```python
from build123d import *

# Parameters (mm, degrees)
SKETCH1_W           = 40.2
SKETCH1_H           = 61.1
BOSS_EXTRUDE1_DEPTH = 41
CHAMFER1_SIZE       = 1
CHAMFER2_SIZE       = 1
SKETCH2_R           = 5
BOSS_EXTRUDE2_DEPTH = 1


with BuildPart() as part:
    # Sketch1 → Boss-Extrude1 (new body)
    with BuildSketch(Plane(origin=(0, 0, 0), x_dir=(1, 0, 0), z_dir=(0, 1, 0))):
        with Locations((20.1, 30.55)):
            Rectangle(SKETCH1_W, SKETCH1_H)
    extrude(amount=BOSS_EXTRUDE1_DEPTH)

    # Chamfer1
    chamfer1_edges = [part.edges().sort_by_distance(p)[0] for p in [
        (40.2, 41, -30.55),
        (20.1, 41, -61.1),
        (0, 41, -30.55),
        (20.1, 41, 0),
    ]]
    chamfer(chamfer1_edges, length=CHAMFER1_SIZE)

    # Chamfer2
    chamfer2_edges = [part.edges().sort_by_distance(p)[0] for p in [
        (20.1, 0, -61.1),
        (40.2, 0, -30.55),
        (20.1, 0, 0),
        (0, 0, -30.55),
    ]]
    chamfer(chamfer2_edges, length=CHAMFER2_SIZE)

    # Sketch2 → Boss-Extrude2 (add)
    with BuildSketch(Plane.XZ):
        with Locations(Location((20.1, -17.640972678, 0), (0, 0, 90))):
            Circle(SKETCH2_R)
    boss_extrude2 = extrude(amount=BOSS_EXTRUDE2_DEPTH)

    # Mirror1: Boss-Extrude2 across plane
    add(boss_extrude2.mirror(Plane.ZX.offset(20.5)))


solid = part.part
```
The model under review builds one solid part; all positions refer to its coordinate system, in mm. A direction names the side the tool comes from. Give positions to 0.01 mm unless a question says otherwise; leave off trailing zeros. Write each loop counter-clockwise with the first axis right and the second up, starting at its lowest first coordinate (ties: lowest second). Pieces come first, ordered by that corner, then holes.
(1) The part is to be moulded in two halves that separate along X. For faces 3 (the flat face through (20, 42, -18)), 4 (the cylindrical face through (19.88, -0.493, -22.636)), 5 (the flat face through (40.2, 20, -30)), 6 (the flat face through (0, 20, -30)), say which applies: released by +X, released by -X, zero draft, split by the parting line, or undercut.
(2) Consider section B-B, the plane x = 4. Give the boundary of the cut face in (y, z).
(3) Consider section C-C, the plane x = 20.1. Give the boundary of the cut face in (y, z), and give its area (3 significant figures).
(4) For P1, Ø1, axis at x = 25.5, z = -44.5, coming from the -Y side, flat-tipped, find the tip position at first contact; note if it passes through.
(5) Consider section D-D, the plane z = -13.5. Give the boundary of the cut face in (x, y).
(6) To check wall thickness, follow L1, parallel to Y at x = 8.5, z = -24.5. State the ranges of the line that lie inside material, in increasing order.
(7) Tool access review of faces 1 (the flat face through (20, 20, -61.1)), 2 (the cylindrical face through (19.88, 41.493, -22.636)): name each direction out of +Z, -Z, +X, -X, +Y, -Y from which nothing blocks a thin tool from reaching the whole face with its end or side.
(8) Consider section A-A, the plane z = -31.5. Give the boundary of the cut face in (x, y).
Returned:
1. face 3: zero draft
1. face 4: split by the parting line
1. face 5: released by +X
1. face 6: released by -X
2. outline: (0, -60.1) - (1, -61.1) - (40, -61.1) - (41, -60.1) - (41, -1) - (40, 0) - (1, 0) - (0, -1) - close
3. outline: (-1, -22.64) - (0, -22.64) - (0, -60.1) - (1, -61.1) - (40, -61.1) - (41, -60.1) - (41, -22.64) - (42, -22.64) - (42, -12.64) - (41, -12.64) - (41, -1) - (40, 0) - (1, 0) - (0, -1) - (0, -12.64) - (-1, -12.64) - close
3. area: 2,520 mm2
4. P1: stops at y = 0
5. outline: (0, 1) - (1, 0) - (17.3, 0) - (17.3, -1) - (22.9, -1) - (22.9, 0) - (39.2, 0) - (40.2, 1) - (40.2, 40) - (39.2, 41) - (22.9, 41) - (22.9, 42) - (17.3, 42) - (17.3, 41) - (1, 41) - (0, 40) - close
6. L1: y = 0 to 41
7. face 1: -Z, +X, -X, +Y, -Y
7. face 2: +Y
8. outline: (0, 1) - (1, 0) - (39.2, 0) - (40.2, 1) - (40.2, 40) - (39.2, 41) - (1, 41) - (0, 40) - close
